Read the model definition and answer for the solid it produces. Units are mm, in the model's axes. Face numbers are marked on the shaded views. Coordinates: 2 decimals unless noted, no trailing zeros. Order: outer loops, then holes, each group sorted by start corner. A loop starts at its lowest first (then second) coordinate and runs counter-clockwise, first axis right, second up. Notation, with made-up numbers: (62, 72.5) -> (68, 72.5) arc R30 cw to (68, 99.5) -> close; hole circle Ø3 at (45.25, 41.25). An arc over 180 degrees is marked (long way). Answer as a JSON object with one key per item and string values. Group by question number.
1) Determine the mould class of the marked faces 1, 2, 3 and 4 for opening direction Z: released by +Z, released by -Z, zero draft, split by the parting line, or undercut.
2) Section A-A on x = 13.25 is taken. Determine the outline of the cut face in (y, z), and give its area (3 significant figures).
3) Consider L1, parallel to X at y = 0.1, z = -2.7; L2, parallel to Z at x = 3.25, y = 0.5; L3, parallel to X at y = 0.35, z = -1.9. Determine where each line is inside the solid, lowest interval first.
4) Section C-C on y = 0.7 is taken. Determine the outline of the cut face in (x, z), and give its area (3 significant figures).
5) Section B-B on z = -2.8 is taken. Determine the outline of the cut face in (x, y), and give its area (3 significant figures).
6) Given pin 1 (3 mm diameter, centred on x = 13.25, z = -2.8, fed in from +Y), flat-ended and moving along its own axis, determine where the tip first touches the part or whether it passes through.
from build123d import *

# Parameters (mm, degrees)
SKETCH1_W                 = 16.5
SKETCH1_H                 = 5.6
BOSS_EXTRUDE1_DEPTH       = 1
M3X0_5_TAPPED_HOLE3_D     = 2.5
M3X0_5_TAPPED_HOLE3_DEPTH = 1


with BuildPart() as part:
    # Sketch1 → Boss-Extrude1 (new body)
    with BuildSketch(Plane(origin=(0, 0, 0), x_dir=(1, 0, 0), z_dir=(0, 1, 0))):
        with Locations((8.25, 2.8)):
            Rectangle(SKETCH1_W, SKETCH1_H)
    extrude(amount=BOSS_EXTRUDE1_DEPTH)

    # M3x0.5 Tapped Hole3
    with Locations(Plane(origin=(0, 1, 0), x_dir=(-1, 0, 0), z_dir=(0, 1, 0))):
        with Locations((-3.25, -2.8), (-13.25, -2.8)):
            Hole(M3X0_5_TAPPED_HOLE3_D / 2, depth=M3X0_5_TAPPED_HOLE3_DEPTH)


solid = part.part
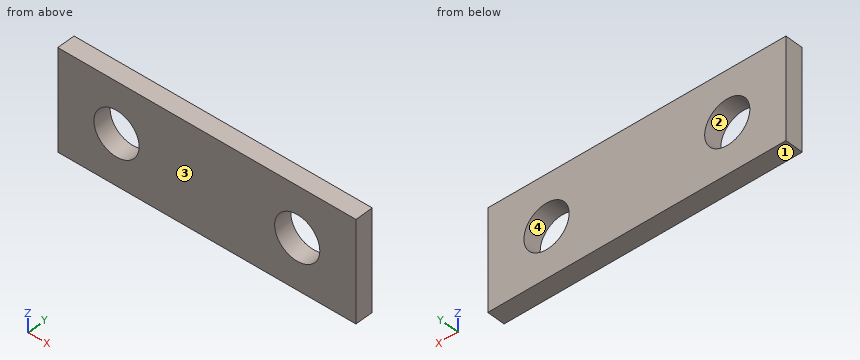
Worked answers:
{
 "1": {"face 1": "released by -Z", "face 2": "undercut", "face 3": "zero draft", "face 4": "undercut"},
 "2": {"outline": "(0, -5.6) -> (1, -5.6) -> (1, -4.05) -> (0, -4.05) -> close; (0, -1.55) -> (1, -1.55) -> (1, 0) -> (0, 0) -> close", "area": "3.10 mm²"},
 "3": {"L1": "x = 0 to 2, 4.5 to 12, 14.5 to 16.5", "L2": "z = -5.6 to -4.05, -1.55 to 0", "L3": "x = 0 to 2.38, 4.12 to 12.38, 14.12 to 16.5"},
 "4": {"outline": "(0, -5.6) -> (16.5, -5.6) -> (16.5, 0) -> (0, 0) -> close; hole circle Ø2.5 at (3.25, -2.8); hole circle Ø2.5 at (13.25, -2.8)", "area": "82.6 mm²"},
 "5": {"outline": "(0, 0) -> (2, 0) -> (2, 1) -> (0, 1) -> close; (4.5, 0) -> (12, 0) -> (12, 1) -> (4.5, 1) -> close; (14.5, 0) -> (16.5, 0) -> (16.5, 1) -> (14.5, 1) -> close", "area": "11.5 mm²"},
 "6": {"pin 1": "stops at y = 1"}
}
